Autodesk Fusion 360 part; units mm, degrees
sketch "Sketch1" plane through (0, 0, 0) normal (0, 0, 1) x (1, 0, 0)
  circle A0 centre (0, 0) radius 13.5
  circle A1 centre (0, 0) radius 15.5
  line L0 (0, 0) -> (-5.3013, 14.5652)
  line L1 (0, 0) -> (5.3013, 14.5652)
  line L2 (0, 0) -> (0, 25)
  dimension "d1" = 27
  dimension "d2" = 31
  dimension "d3" = 20
  dimension "d4" = 20
extrude "Extrude1" add sketch "Sketch1" along normal blind 12 contours A0 A1 L0 L1
fillet "Fillet1" radius 1 4 edges at (-5.3013, 14.5652, 6) (-4.6173, 12.6859, 6) (4.6173, 12.6859, 6) (5.3013, 14.5652, 6)
equation "d2 = d1 + 4 mm"
equation "d4 = d3"
The listing builds one solid part. Answer for the finished solid, in the listing's coordinates (mm). A direction names the side the tool comes from. Give positions to 0.01 mm unless a question says otherwise; leave off trailing zeros. Write each loop counter-clockwise with the first axis right and the second up, starting at its lowest first coordinate (ties: lowest second). Pieces come first, ordered by that corner, then holes. Notation, with made-up numbers: (-13, -15.75) -> (-3, -15.75) arc R20 ccw to (-3, 3.25) -> close; hole circle Ø3 at (34.25, 57). An arc over 180 degrees is marked (long way). Write item = value, one per line. Start each with the question number.
1) The part is cut by section B-B, the plane x = -8. Determine the outline of the cut face in (y, z).
2) Straight lines are drawn through the part: line 1 along X through (y, z) = (0, 3.75); line 2 along Y through (x, z) = (0, 7); line 3 along X through (y, z) = (7.75, 1.5). For each, find the intervals that lie inside material, in ascending order.
3) Which of the six approach directions +Z, -Z, +X, -X, +Y, -Y give full straight-line access (tool end or side, diameter ignored) to faces 1 (the face through (-4.97, 12.85, 6.08)), 2 (the face through (-5.49, 14.17, 6.08))?
4) Each of these flat-tipped pins is pushed along its axis until it touches: pin 1 (2 mm diameter, centred on x = -2, z = 7, fed in from +Y); pin 2 (1.5 mm diameter, centred on x = 11.5, y = 4.5, fed in from +Z); pin 3 (1 mm diameter, centred on x = 11.5, z = 8, fed in from -Y). Where does it stop, or does it pass through?
5) The part is cut by section A-A, the plane y = 0. Determine the outline of the cut face in (x, z).
6) The part is cut by section D-D, the plane x = 0. Determine the outline of the cut face in (y, z), and give its area (3 significant figures).
7) Determine the mould class of faces 3 (the face through (0.59, -15.49, 5.92)), 4 (the face through (-5, -13, 0)), 5 (the face through (4.963, 12.87, 6.084)) for opening direction X: +X half, -X half, draft (parallel to the pull), parting line (faces both ways), or undercut.
Solutions:
q1.outline = (-13.28, 0) -> (-10.87, 0) -> (-10.87, 12) -> (-13.28, 12) -> close; (10.87, 0) -> (13.28, 0) -> (13.28, 12) -> (10.87, 12) -> close
q2.line_1 = -15.5 to -13.5, 13.5 to 15.5
q2.line_2 = -15.5 to -13.5
q2.line_3 = -13.42 to -11.05, 11.05 to 13.42
q3.face_1 = +Z, -Z
q3.face_2 = +Z, -Z, +Y
q4.pin_1 = -13.16
q4.pin_2 = through
q4.pin_3 = -10.92
q5.outline = (-15.5, 0) -> (-13.5, 0) -> (-13.5, 12) -> (-15.5, 12) -> close; (13.5, 0) -> (15.5, 0) -> (15.5, 12) -> (13.5, 12) -> close
q6.outline = (-15.5, 0) -> (-13.5, 0) -> (-13.5, 12) -> (-15.5, 12) -> close
q6.area = 24.0 mm²
q7.face_3 = parting line
q7.face_4 = draft
q7.face_5 = undercut
